```python
from build123d import *

# Parameters (mm, degrees)
SKETCH1_R           = 2.15
BOSS_EXTRUDE1_DEPTH = 3.175


with BuildPart() as part:
    # Sketch1 → Boss-Extrude1 (new body)
    with BuildSketch(Plane(origin=(0, 0, 0), x_dir=(1, 0, 0), z_dir=(0, 1, 0))):
        with BuildLine():
            Line((98.331536726, 6.35), (-9.431536726, 6.35))
            ThreePointArc((-9.431536726, 6.35), (-11.861576522, 5.866635031), (-13.921664787, 4.490128061))
            Line((-13.921664787, 4.490128061), (-49.842689271, -31.430896424))
            ThreePointArc((-49.842689271, -31.430896424), (-51.409271688, -37.828577417), (-46.459210265, -42.173850075))
            Line((-46.459210265, -42.173850075), (-13.806649055, -47.952825591))
            ThreePointArc((-13.806649055, -47.952825591), (-13.255453642, -48.025659748), (-12.7, -48.05))
            Line((-12.7, -48.05), (101.6, -48.05))
            ThreePointArc((101.6, -48.05), (102.155453642, -48.025659748), (102.706649055, -47.952825591))
            Line((102.706649055, -47.952825591), (135.359210265, -42.173850075))
            ThreePointArc((135.359210265, -42.173850075), (140.309271688, -37.828577417), (138.742689271, -31.430896424))
            Line((138.742689271, -31.430896424), (102.821664787, 4.490128061))
            ThreePointArc((102.821664787, 4.490128061), (100.761576522, 5.866635031), (98.331536726, 6.35))
        make_face()
        with Locations(Location((0, 0, 0), (0, 0, 270))):
            Circle(SKETCH1_R, mode=Mode.SUBTRACT)
        with Locations(Location((25.4, 0, 0), (0, 0, 270))):
            Circle(SKETCH1_R, mode=Mode.SUBTRACT)
        with Locations(Location((-18.411792847, -8.980256121, 0), (0, 0, 270))):
            Circle(SKETCH1_R, mode=Mode.SUBTRACT)
        with Locations(Location((-27.392048969, -17.960512242, 0), (0, 0, 270))):
            Circle(SKETCH1_R, mode=Mode.SUBTRACT)
        with Locations(Location((-36.37230509, -26.940768363, 0), (0, 0, 270))):
            Circle(SKETCH1_R, mode=Mode.SUBTRACT)
        with Locations(Location((-45.352561211, -35.921024484, 0), (0, 0, 270))):
            Circle(SKETCH1_R, mode=Mode.SUBTRACT)
        with Locations(Location((-12.7, -41.7, 0), (0, 0, 270))):
            Circle(SKETCH1_R, mode=Mode.SUBTRACT)
        with Locations(Location((12.7, -41.7, 0), (0, 0, 270))):
            Circle(SKETCH1_R, mode=Mode.SUBTRACT)
        with Locations(Location((63.5, 0, 0), (0, 0, 90))):
            Circle(SKETCH1_R, mode=Mode.SUBTRACT)
        with Locations(Location((88.9, 0, 0), (0, 0, 90))):
            Circle(SKETCH1_R, mode=Mode.SUBTRACT)
        with Locations(Location((107.311792847, -8.980256121, 0), (0, 0, 90))):
            Circle(SKETCH1_R, mode=Mode.SUBTRACT)
        with Locations(Location((116.292048969, -17.960512242, 0), (0, 0, 90))):
            Circle(SKETCH1_R, mode=Mode.SUBTRACT)
        with Locations(Location((134.252561211, -35.921024484, 0), (0, 0, 90))):
            Circle(SKETCH1_R, mode=Mode.SUBTRACT)
        with Locations(Location((125.27230509, -26.940768363, 0), (0, 0, 90))):
            Circle(SKETCH1_R, mode=Mode.SUBTRACT)
        with Locations(Location((76.2, -41.7, 0), (0, 0, 90))):
            Circle(SKETCH1_R, mode=Mode.SUBTRACT)
        with Locations(Location((101.6, -41.7, 0), (0, 0, 90))):
            Circle(SKETCH1_R, mode=Mode.SUBTRACT)
        with BuildLine():
            Line((95.25, -6.35), (-6.35, -6.35))
            ThreePointArc((-6.35, -6.35), (-10.840128061, -8.209871939), (-12.7, -12.7))
            Line((-12.7, -12.7), (-12.7, -29))
            ThreePointArc((-12.7, -29), (-10.840128061, -33.490128061), (-6.35, -35.35))
            Line((-6.35, -35.35), (95.25, -35.35))
            ThreePointArc((95.25, -35.35), (99.740128061, -33.490128061), (101.6, -29))
            Line((101.6, -29), (101.6, -12.7))
            ThreePointArc((101.6, -12.7), (99.740128061, -8.209871939), (95.25, -6.35))
        make_face(mode=Mode.SUBTRACT)
    extrude(amount=BOSS_EXTRUDE1_DEPTH)


solid = part.part
```
Input: part model. Units: mm. Frame: model coordinates. A direction names the side the tool comes from. Coordinates: 2 decimals unless noted, no trailing zeros. Write each loop counter-clockwise with the first axis right and the second up, starting at its lowest first coordinate (ties: lowest second). Pieces come first, ordered by that corner, then holes. Notation, with made-up numbers: (44.25, -3.75) -> (80.25, -3.75) arc R21 ccw to (80.25, 3.25) -> close; hole circle Ø6 at (-0.5, -34). An arc over 180 degrees is marked (long way). Answer as a JSON object with one key per item and string values.
1. Material intervals for line 1 (Z direction, x = 63.5, y = 1.25); line 2 (Z direction, x = 18, y = 2.15); line 3 (X direction, y = 1.5, z = 25), sorted ascending. Write a range as from..to.
Result set:
{"line 1": "z = -6.35..-2.15, 2.15..6.35, 35.35..48.05", "line 2": "z = -6.35..6.35, 35.35..48.05", "line 3": "x = -43.41..-37.3, -35.45..-12.7, 101.6..124.35, 126.2..132.31"}
2. Section C-C on z = 0. Return the cut outline in (x, y) (3 decimals).
Result set:
{"outline": "(-18.412, 0) -> (-2.15, 0) -> (-2.15, 3.175) -> (-18.412, 3.175) -> close; (2.15, 0) -> (23.25, 0) -> (23.25, 3.175) -> (2.15, 3.175) -> close; (27.55, 0) -> (61.35, 0) -> (61.35, 3.175) -> (27.55, 3.175) -> close; (65.65, 0) -> (86.75, 0) -> (86.75, 3.175) -> (65.65, 3.175) -> close; (91.05, 0) -> (107.312, 0) -> (107.312, 3.175) -> (91.05, 3.175) -> close"}
3. First-contact query: P1, Ø1, axis at y = 2, z = 2, coming from the -X side. Flat tip, straight axial feed; report the tip coordinate or a pass-through.
Result set:
{"P1": "stops at x = -20.91"}
4. Access query for faces 5 (the face through (121.03, 1.57, 13.72)), 6 (the face through (-12.7, 2, 21)). Directions: +Z, -Z, +X, -X, +Y, -Y. A direction counts if a zero-diameter tool reaches every point of the face in a straight line with its end or side. Return the directions, or none.
Result set:
{"face 5": "-Z, +X, +Y, -Y", "face 6": "+Y, -Y"}
5. Section D-D on y = 1.85. Count the separate pieces of the cut face and the enclosed holes in it, then the cut area to 3 significant figures.
Result set:
{"separate pieces": "1", "enclosed holes": "17", "area": "5,100 mm2"}
6. Mould query, pull axis X, two halves, no side actions, for faces 1 (the face through (43, 3.175, 39)), 2 (the face through (100.794, 1.565, -5.853)), 3 (the face through (90.81, 1.57, -0.99)), 4 (the face through (-19.235, 1.565, 10.966)). Classes: released by +X, released by -X, zero draft, split by the parting line, or undercut.
Result set:
{"face 1": "zero draft", "face 2": "released by +X", "face 3": "undercut", "face 4": "undercut"}
7. Section B-B on x = 12.7. Return the cut outline in (y, z) (3 decimals), then the cut area to 3 significant figures.
Result set:
{"outline": "(0, -6.35) -> (3.175, -6.35) -> (3.175, 6.35) -> (0, 6.35) -> close; (0, 35.35) -> (3.175, 35.35) -> (3.175, 39.55) -> (0, 39.55) -> close; (0, 43.85) -> (3.175, 43.85) -> (3.175, 48.05) -> (0, 48.05) -> close", "area": "67.0 mm2"}
8. Section A-A on x = 32.5. Return the cut outline in (y, z) (3 decimals).
Result set:
{"outline": "(0, -6.35) -> (3.175, -6.35) -> (3.175, 6.35) -> (0, 6.35) -> close; (0, 35.35) -> (3.175, 35.35) -> (3.175, 48.05) -> (0, 48.05) -> close"}
